Autodesk Inventor part; units mm, degrees
ref_plane "YZ Plane" through (0, 0, 0) normal (1, 0, 0) x (0, 1, 0)
ref_plane "XZ Plane" through (0, 0, 0) normal (0, 1, 0) x (-1, 0, 0)
ref_plane "XY Plane" through (0, 0, 0) normal (0, 0, 1) x (1, 0, 0)
sketch "Sketch1" plane through (0, 0, 0) normal (0, 0, 1) x (1, 0, 0)
  line L0 (0, 6.9282) -> (6, 3.4641)
  line L1 (6, 3.4641) -> (6, -3.4641)
  line L2 (6, -3.4641) -> (0, -6.9282)
  line L3 (0, -6.9282) -> (-6, -3.4641)
  line L4 (-6, -3.4641) -> (-6, 3.4641)
  line L5 (-6, 3.4641) -> (0, 6.9282)
  point P0 (0, 0)
  point P1 (0, 0)
  point P2 (-6, 0)
  dimension "d0" = 12
extrude "Extrusion1" add sketch "Sketch1" along normal blind 8
chamfer "Chamfer1" distance 1 angle 45 6 edges at (-3, 5.1962, 8) (3, 5.1962, 8) (6, 0, 8) (3, -5.1962, 8) (-3, -5.1962, 8) (-6, 0, 8)
sketch "Sketch2" plane through (0, 0, 8) normal (0, 0, 1) x (1, 0, 0)
  point P0 (0, 0)
  point P1 (0, 0)
hole "Hole1" at (0, 0, 8) direction (0, 0, -1) diameter 6 depth 1.5
sketch "Sketch3" plane through (0, 0, 0) normal (0, 0, -1) x (-1, 0, 0)
  point P0 (0, 0)
  point P1 (0, 0)
hole "Hole2" at (0, 0, 0) direction (0, 0, 1) diameter 6.647 depth 6.5
properties part number "50" material "Steel, Alloy"
Can you work these out from the model? Positions are in its coordinate system, mm. A direction names the side the tool comes from. Coordinates: 2 decimals unless noted, no trailing zeros. Loops run counter-clockwise (first coordinate to the right, second up) from the corner with the lowest first, then second, coordinate; pieces in that order, holes last. Notation, with made-up numbers: (72, -13.5) - (119, -13.5) arc R18 ccw to (119, 4.5) - close; hole circle Ø11 at (-27, 8). An arc over 180 degrees is marked (long way). Put each result on its own line as item: value. Start each with the question number.
Item 1: Suppose I cut it at D-D (y = 6). Please give me the cut outline in (x, z), and give its area (3 significant figures).
Item 2: Suppose I cut it at A-A (z = 1.5). Please give me the cut outline in (x, y).
Item 3: Suppose I cut it at C-C (y = 1.5). Please give me the cut outline in (x, z).
Item 4: Which directions (+Z, -Z, +X, -X, +Y, -Y) give clear straight access to the entire face, cutting with the end or side of a thin tool? Please do faces 4 (the face through (1.27, 3.07, 3.3)), 5 (the face through (-2.96, -5.22, 3.45)).
Item 5: Suppose I cut it at B-B (x = 0.5). Please give me the cut outline in (y, z), and give its area (3 significant figures).
Item 6: If I drill on line 1 along X through (y, z) = (0, 3.75); line 2 along X through (y, z) = (2.75, 1); line 3 along Y through (x, z) = (-2, 4.25), over which ranges is the centre line in solid material (lowest first)?
Item 7: For pin 1 (2 mm diameter, centred on x = 4, y = -5.5, fed in from +Z); pin 2 (2 mm diameter, centred on x = 3, y = -2, fed in from -Z); pin 3 (1 mm diameter, centred on x = -3, z = 1, fed in from +Y), each with a flat end and sliding along its axis, tell me the tip position at first contact or that it passes through.
Item 8: If we mould it in two halves opening along Y, with no side actions, what happens to faces 1 (the face through (-5.5, 0, 7.5)), 2 (the face through (3.042, -5.172, 3.451)), 3 (the face through (0, 3, 7))? For each: +Y half, -Y half, draft (parallel to the pull), parting line (faces both ways), or undercut.
Here are the results:
1. outline: (-1.61, 0) - (1.61, 0) - (1.61, 7) - (0, 7.8) - (-1.61, 7) - close
1. area: 23.8 mm²
2. outline: (-6, -3.46) - (0, -6.93) - (6, -3.46) - (6, 3.46) - (0, 6.93) - (-6, 3.46) - close; hole circle Ø6.65 at (0, 0)
3. outline: (-6, 0) - (-2.97, 0) - (-2.97, 6.5) - (-2.6, 6.5) - (-2.6, 8) - (-5, 8) - (-6, 7) - close; (2.6, 6.5) - (2.97, 6.5) - (2.97, 0) - (6, 0) - (6, 7) - (5, 8) - (2.6, 8) - close
4. face 4: -Z
4. face 5: +Z, -Z, -X, -Y
5. outline: (-6.64, 0) - (-3.29, 0) - (-3.29, 6.5) - (-2.96, 6.5) - (-2.96, 8) - (-5.48, 8) - (-6.64, 7) - close; (2.96, 6.5) - (3.29, 6.5) - (3.29, 0) - (6.64, 0) - (6.64, 7) - (5.48, 8) - (2.96, 8) - close
5. area: 53.5 mm²
6. line 1: -6 to -3.32, 3.32 to 6
6. line 2: -6 to -1.87, 1.87 to 6
6. line 3: -5.77 to -2.65, 2.65 to 5.77
7. pin 1: z = 7.24
7. pin 2: z = 0
7. pin 3: y = 5.48
8. face 1: draft
8. face 2: -Y half
8. face 3: undercut
